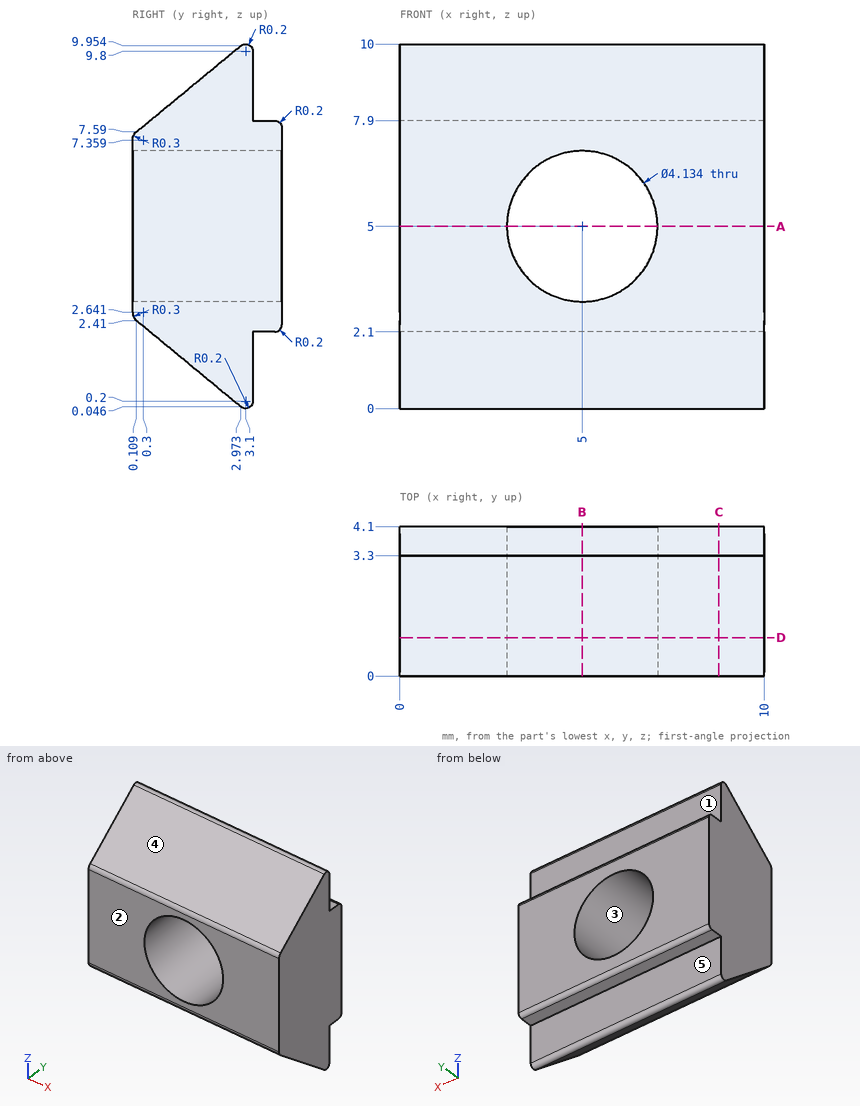
Verification items for this drawing (mm, ordinates from the low corner). A direction names the side the tool comes from. Give positions to 0.01 mm unless a question says otherwise; leave off trailing zeros. Write each loop counter-clockwise with the first axis right and the second up, starting at its lowest first coordinate (ties: lowest second). Pieces come first, ordered by that corner, then holes.
1) Section check D-D, the plane y = 1.05. Record the boundary of the cut face in (x, z).
2) Section check A-A, the plane z = 5. Record the boundary of the cut face in (x, y).
3) Section check C-C, the plane x = 8.75. Record the boundary of the cut face in (y, z), and give its area (3 significant figures).
4) Access from +Z, -Z, +X, -X, +Y, -Y to the whole of each face (thin tool, end or side, straight path). Record for the marked faces 1 and 2.
5) Material ranges on L1, parallel to X at y = 3.3, z = 6.5; L2, parallel to Z at x = 5, y = 1.8 (1 decimal); L3, parallel to Z at x = 5, y = 2, recorded low to high.
6) Gauge pin test, flat ends, axial feed: pin 1 (2 mm diameter, centred on x = 7, z = 1, fed in from +Y); pin 2 (0.7 mm diameter, centred on x = 4, y = 3.5, fed in from +Z); pin 3 (3 mm diameter, centred on x = 2, z = 8, fed in from -Y). Record the tip position at first contact, or that the pin passes through.
7) Release check for a two-part mould opening along Z. For the marked faces 3, 4 and 5 record: pulls with the +Z half, pulls with the -Z half, needs draft (parallel to the pull), parting line crosses it, or undercut.
8) Section check B-B, the plane x = 5. Record the boundary of the cut face in (y, z).
Computed:
1. outline: (0, 1.63) - (10, 1.63) - (10, 8.37) - (0, 8.37) - close; hole circle Ø4.13 at (5, 5)
2. outline: (0, 0) - (2.93, 0) - (2.93, 4.1) - (0, 4.1) - close; (7.07, 0) - (10, 0) - (10, 4.1) - (7.07, 4.1) - close
3. outline: (0, 2.64) arc R0.3 ccw to (0.11, 2.41) - (2.97, 0.05) arc R0.2 ccw to (3.3, 0.2) - (3.3, 2.1) - (3.9, 2.1) arc R0.2 ccw to (4.1, 2.3) - (4.1, 7.7) arc R0.2 ccw to (3.9, 7.9) - (3.3, 7.9) - (3.3, 9.8) arc R0.2 ccw to (2.97, 9.95) - (0.11, 7.59) arc R0.3 ccw to (0, 7.36) - close
3. area: 30.0 mm2
4. face 1: +Z, +X, -X, +Y
4. face 2: +Z, -Z, +X, -X, -Y
5. L1: x = 0 to 3.58, 6.42 to 10
5. L2: z = 1 to 2.9, 7.1 to 9
5. L3: z = 0.85 to 2.93, 7.07 to 9.15
6. pin 1: stops at y = 3.3
6. pin 2: stops at z = 9.99
6. pin 3: stops at y = 0
7. face 3: undercut
7. face 4: pulls with the +Z half
7. face 5: needs draft
8. outline: (0, 2.64) arc R0.3 ccw to (0.11, 2.41) - (2.97, 0.05) arc R0.2 ccw to (3.3, 0.2) - (3.3, 2.1) - (3.9, 2.1) arc R0.2 ccw to (4.1, 2.3) - (4.1, 2.93) - (0, 2.93) - close; (0, 7.07) - (4.1, 7.07) - (4.1, 7.7) arc R0.2 ccw to (3.9, 7.9) - (3.3, 7.9) - (3.3, 9.8) arc R0.2 ccw to (2.97, 9.95) - (0.11, 7.59) arc R0.3 ccw to (0, 7.36) - close
